from build123d import *

# Parameters (mm, degrees)
CIRPATTERN2_COUNT              = 3
F_50_0_07_DIAMETER_HOLE1_D     = 1.778
F_50_0_07_DIAMETER_HOLE1_DEPTH = 11.938
F_50_0_07_DIAMETER_HOLE1_TIP   = 0.53416509
SKETCH60_R                     = 4.7625
BOSS_EXTRUDE4_DEPTH            = 5.461
CUT_EXTRUDE1_REACH             = 51.399
SKETCH54_R                     = 0.80645
F_1_16_0_0625_DIAMETER_HOLE1_D = 1.5875
Q_0_332_DIAMETER_HOLE2_D       = 8.4328
Q_0_332_DIAMETER_HOLE2_DEPTH   = 8.89
Q_0_332_DIAMETER_HOLE2_TIP     = 2.533468714


with BuildPart() as part:
    # Sketch1 → Revolve1 (revolve)
    with BuildSketch(Plane.XY, mode=Mode.PRIVATE) as revolve1_sk:
        Polygon((-12.599, 0), (0, 0), (0, 32.512), (-2.54, 32.512), (-2.54, 30.48), (-6.223, 30.48), (-6.223, 32.512), (-8.763, 32.512), (-8.763, 30.48), (-12.446, 30.48), (-12.446, 32.512), (-14.885, 32.512), (-14.885, 29.1592), (-18.06, 29.1592), (-18.06, 4.7625), (-12.599, 4.7625), align=None)
    revolve(revolve1_sk.sketch.rotate(Axis((17.779879847, 0, 0), (-1, 0, 0)), 90), axis=Axis((17.779879847, 0, 0), (-1, 0, 0)))

    # Sketch24 → #20 (0.161) Diameter Hole1 (revolve, cut)
    with BuildSketch(Plane(origin=(-18.06, 20.6375, 0), x_dir=(0, 0, 1), z_dir=(0, 1, 0))):
        Polygon((0, 0), (0, 10.880579708), (2.0447, 9.652), (2.0447, 0), align=None)
    f_20_0_161_diameter_hole1 = revolve(axis=Axis((-24.41, 20.6375, 0), (1, 0, 0)), mode=Mode.SUBTRACT)

    # CirPattern2: #20 (0.161) Diameter Hole1 ×3 about axis
    cirpattern2_axis = Axis((0, 0, 0), (1, 0, 0))
    for i in range(1, CIRPATTERN2_COUNT):
        add(f_20_0_161_diameter_hole1.rotate(cirpattern2_axis, i * 360 / CIRPATTERN2_COUNT), mode=Mode.SUBTRACT)

    # #50 (0.07) Diameter Hole1
    with Locations(Plane.ZY.offset(18.06)):
        with Locations((17.872599271, 10.31875)):
            Hole(F_50_0_07_DIAMETER_HOLE1_D / 2, depth=F_50_0_07_DIAMETER_HOLE1_DEPTH)
            with Locations((0, 0, -(F_50_0_07_DIAMETER_HOLE1_DEPTH + F_50_0_07_DIAMETER_HOLE1_TIP / 2))):  # 118° drill point
                Cone(0, F_50_0_07_DIAMETER_HOLE1_D / 2, F_50_0_07_DIAMETER_HOLE1_TIP, mode=Mode.SUBTRACT)

    # Sketch60 → Boss-Extrude4 (add)
    with BuildSketch(Plane.ZY.offset(12.599)):
        Circle(SKETCH60_R)
    extrude(amount=BOSS_EXTRUDE4_DEPTH)

    # Sketch54 → Cut-Extrude1 (cut, up to next)
    with BuildSketch(Plane(origin=(0, 0, 0), x_dir=(0, 0, -1), z_dir=(1, 0, 0)), mode=Mode.PRIVATE) as cut_extrude1_sk1:
        with Locations((0, 6.477)):
            Circle(SKETCH54_R)
    cut_extrude1_tool1 = extrude(cut_extrude1_sk1.sketch, amount=-CUT_EXTRUDE1_REACH, mode=Mode.PRIVATE) & part.part
    # Sketch54 → Cut-Extrude1 (cut, up to next)
    with BuildSketch(Plane(origin=(0, 0, 0), x_dir=(0, 0, -1), z_dir=(1, 0, 0)), mode=Mode.PRIVATE) as cut_extrude1_sk2:
        with Locations((4.579930622, 4.579930622)):
            Circle(SKETCH54_R)
    cut_extrude1_tool2 = extrude(cut_extrude1_sk2.sketch, amount=-CUT_EXTRUDE1_REACH, mode=Mode.PRIVATE) & part.part
    # Sketch54 → Cut-Extrude1 (cut, up to next)
    with BuildSketch(Plane(origin=(0, 0, 0), x_dir=(0, 0, -1), z_dir=(1, 0, 0)), mode=Mode.PRIVATE) as cut_extrude1_sk3:
        with Locations((6.477, 0)):
            Circle(SKETCH54_R)
    cut_extrude1_tool3 = extrude(cut_extrude1_sk3.sketch, amount=-CUT_EXTRUDE1_REACH, mode=Mode.PRIVATE) & part.part
    # Sketch54 → Cut-Extrude1 (cut, up to next)
    with BuildSketch(Plane(origin=(0, 0, 0), x_dir=(0, 0, -1), z_dir=(1, 0, 0)), mode=Mode.PRIVATE) as cut_extrude1_sk4:
        with Locations((4.579930622, -4.579930622)):
            Circle(SKETCH54_R)
    cut_extrude1_tool4 = extrude(cut_extrude1_sk4.sketch, amount=-CUT_EXTRUDE1_REACH, mode=Mode.PRIVATE) & part.part
    # Sketch54 → Cut-Extrude1 (cut, up to next)
    with BuildSketch(Plane(origin=(0, 0, 0), x_dir=(0, 0, -1), z_dir=(1, 0, 0)), mode=Mode.PRIVATE) as cut_extrude1_sk5:
        with Locations((0, -6.477)):
            Circle(SKETCH54_R)
    cut_extrude1_tool5 = extrude(cut_extrude1_sk5.sketch, amount=-CUT_EXTRUDE1_REACH, mode=Mode.PRIVATE) & part.part
    # Sketch54 → Cut-Extrude1 (cut, up to next)
    with BuildSketch(Plane(origin=(0, 0, 0), x_dir=(0, 0, -1), z_dir=(1, 0, 0)), mode=Mode.PRIVATE) as cut_extrude1_sk6:
        with Locations((-4.579930622, -4.579930622)):
            Circle(SKETCH54_R)
    cut_extrude1_tool6 = extrude(cut_extrude1_sk6.sketch, amount=-CUT_EXTRUDE1_REACH, mode=Mode.PRIVATE) & part.part
    # Sketch54 → Cut-Extrude1 (cut, up to next)
    with BuildSketch(Plane(origin=(0, 0, 0), x_dir=(0, 0, -1), z_dir=(1, 0, 0)), mode=Mode.PRIVATE) as cut_extrude1_sk7:
        with Locations((-6.477, 0)):
            Circle(SKETCH54_R)
    cut_extrude1_tool7 = extrude(cut_extrude1_sk7.sketch, amount=-CUT_EXTRUDE1_REACH, mode=Mode.PRIVATE) & part.part
    # Sketch54 → Cut-Extrude1 (cut, up to next)
    with BuildSketch(Plane(origin=(0, 0, 0), x_dir=(0, 0, -1), z_dir=(1, 0, 0)), mode=Mode.PRIVATE) as cut_extrude1_sk8:
        with Locations((-4.579930622, 4.579930622)):
            Circle(SKETCH54_R)
    cut_extrude1_tool8 = extrude(cut_extrude1_sk8.sketch, amount=-CUT_EXTRUDE1_REACH, mode=Mode.PRIVATE) & part.part
    add(cut_extrude1_tool1.solids().sort_by_distance((0, 6.477, 0))[0], mode=Mode.SUBTRACT)
    add(cut_extrude1_tool2.solids().sort_by_distance((0, 4.579931, -4.579931))[0], mode=Mode.SUBTRACT)
    add(cut_extrude1_tool3.solids().sort_by_distance((0, 0, -6.477))[0], mode=Mode.SUBTRACT)
    add(cut_extrude1_tool4.solids().sort_by_distance((0, -4.579931, -4.579931))[0], mode=Mode.SUBTRACT)
    add(cut_extrude1_tool5.solids().sort_by_distance((0, -6.477, 0))[0], mode=Mode.SUBTRACT)
    add(cut_extrude1_tool6.solids().sort_by_distance((0, -4.579931, 4.579931))[0], mode=Mode.SUBTRACT)
    add(cut_extrude1_tool7.solids().sort_by_distance((0, 0, 6.477))[0], mode=Mode.SUBTRACT)
    add(cut_extrude1_tool8.solids().sort_by_distance((0, 4.579931, 4.579931))[0], mode=Mode.SUBTRACT)

    # 1/16 (0.0625) Diameter Hole1 (through all)
    with Locations(Plane(origin=(0, -22.225, 0), x_dir=(0, 0, 1), z_dir=(1, 0, 0))):
        with Locations((0, 0)):
            Hole(F_1_16_0_0625_DIAMETER_HOLE1_D / 2)

    # Q (0.332) Diameter Hole2
    with Locations(Plane(origin=(-18.06, -22.225, 0), x_dir=(0, 0, -1), z_dir=(-1, 0, 0))):
        with Locations((0, 0)):
            Hole(Q_0_332_DIAMETER_HOLE2_D / 2, depth=Q_0_332_DIAMETER_HOLE2_DEPTH)
            with Locations((0, 0, -(Q_0_332_DIAMETER_HOLE2_DEPTH + Q_0_332_DIAMETER_HOLE2_TIP / 2))):  # 118° drill point
                Cone(0, Q_0_332_DIAMETER_HOLE2_D / 2, Q_0_332_DIAMETER_HOLE2_TIP, mode=Mode.SUBTRACT)


solid = part.part
Read the model definition and answer for the solid it produces. Units are mm, in the model's axes. A direction names the side the tool comes from. Coordinates: 2 decimals unless noted, no trailing zeros. Loops run counter-clockwise (first coordinate to the right, second up) from the corner with the lowest first, then second, coordinate; pieces in that order, holes last. Notation, with made-up numbers: (-11.75, 73) - (47.25, 73) arc R18 ccw to (47.25, 82) - close; hole circle Ø8 at (76.25, -9). An arc over 180 degrees is marked (long way). Answer in a Markdown table with one row per item.
Q1. For faces 1 (the cylindrical face through (-13.3, -9.5, -16)), 2 (the flat face through (-6.223, -29, -10)), 3 (the cylindrical face through (-8.904, -5.677, 0.105)), determine the directions among +Z, -Z, +X, -X, +Y, -Y from which every point of the face is accessible in a straight line to the end or side of a thin tool.
Here are the results:
| item | result |
|---|---|
| face 1 | -X |
| face 2 | none |
| face 3 | +X, -X |
Q2. Find section B-B on y = 16.5. Write down the section's boundary in (x, z) (3 decimals), plus the area to 3 significant figures.
Here are the results:
| item | result |
|---|---|
| outline | (-18.06, -24.042) - (-14.885, -24.042) - (-14.885, -28.014) - (-12.446, -28.014) - (-12.446, -25.628) - (-8.763, -25.628) - (-8.763, -28.014) - (-6.223, -28.014) - (-6.223, -25.628) - (-2.54, -25.628) - (-2.54, -28.014) - (0, -28.014) - (0, 28.014) - (-2.54, 28.014) - (-2.54, 25.628) - (-6.223, 25.628) - (-6.223, 28.014) - (-8.763, 28.014) - (-8.763, 25.628) - (-12.446, 25.628) - (-12.446, 28.014) - (-14.885, 28.014) - (-14.885, 24.042) - (-18.06, 24.042) - close |
| area | 951 mm^2 |
Q3. The mould has two halves that part along Z. Classify faces 4 (the cylindrical face through (-8.904, 0.242, -7.246)), 5 (the cylindrical face through (-1.29, 31.74, 7.05)), 6 (the flat face through (-8.763, -29, 10)): pulls with the +Z half, pulls with the -Z half, needs draft (parallel to the pull), parting line crosses it, or undercut.
Here are the results:
| item | result |
|---|---|
| face 4 | undercut |
| face 5 | parting line crosses it |
| face 6 | needs draft |
Q4. Find section A-A on y = 0. Count the separate pieces of the cut face and the enclosed holes in it, plus the area to 3 significant figures.
Here are the results:
| item | result |
|---|---|
| separate pieces | 3 |
| enclosed holes | 0 |
| area | 1,060 mm^2 |
Q5. Straight lines are drawn through the part: line 1 along Y through (x, z) = (-13.5, 0); line 2 along Z through (x, y) = (-7.5, -22); line 3 along Y through (x, z) = (-15.25, -16). For each, find the intervals that lie inside material, in ascending order. Write a range as [from, to].
Here are the results:
| item | result |
|---|---|
| line 1 | y = [-32.51, -26.44], [-18.01, -7.28], [-5.67, 5.67], [7.28, 18.59], [22.68, 32.51] |
| line 2 | z = [-23.94, -1.42], [1.42, 23.94] |
| line 3 | y = [-24.38, -11.14], [-9.5, 24.38] |
Q6. Find section C-C on z = 25. Write down the section's boundary in (x, y) (3 decimals), plus the area to 3 significant figures.
Here are the results:
| item | result |
|---|---|
| outline | (-18.06, -15.009) - (-14.885, -15.009) - (-14.885, -20.785) - (-12.446, -20.785) - (-12.446, -17.436) - (-8.763, -17.436) - (-8.763, -20.785) - (-6.223, -20.785) - (-6.223, -17.436) - (-2.54, -17.436) - (-2.54, -20.785) - (0, -20.785) - (0, 20.785) - (-2.54, 20.785) - (-2.54, 17.436) - (-6.223, 17.436) - (-6.223, 20.785) - (-8.763, 20.785) - (-8.763, 17.436) - (-12.446, 17.436) - (-12.446, 20.785) - (-14.885, 20.785) - (-14.885, 15.009) - (-18.06, 15.009) - close |
| area | 665 mm^2 |
Q7. Given P1, Ø1.5, axis at y = 6.477, z = 0, coming from the +X side; P2, Ø3, axis at x = -15.5, y = 11, coming from the +Z side; P3, Ø2, axis at x = -11, y = -18, coming from the -Z side; P4, Ø1.5, axis at x = -14.5, y = 3.5, coming from the -Z side, each flat-ended and moving along its own axis, determine where each tip first touches the part or whether it passes through.
Here are the results:
| item | result |
|---|---|
| P1 | passes through |
| P2 | stops at z = 31.05 |
| P3 | stops at z = -25.3 |
| P4 | stops at z = -32.4 |
